The figure shows three views and two pictorial views of one solid part (mm, origin at its lowest corner). Answer the questions. A direction names the side the tool comes from. Round coordinates to 2 decimals unless told otherwise and drop trailing zeros. Order: outer loops, then holes, each group sorted by start corner. A loop starts at its lowest first (then second) coordinate and runs counter-clockwise, first axis right, second up. Notation, with made-up numbers: (41, 28.25) - (49, 28.25) arc R22 cw to (49, 56.25) - close; hole circle Ø5 at (47, 82). An arc over 180 degrees is marked (long way). Use CSV: the item, a comma, the result in double quotes. Start each with the question number.
Item 1: Find section D-D, the plane x = 8.5. Give the vertices of the cut face in (y, z), plus the area to 3 significant figures.
Item 2: Straight lines are drawn through the part: line 1 along X through (y, z) = (0.8, 7.5) (3 decimals); line 2 along Y through (x, z) = (3.25, 3.25); line 3 along Y through (x, z) = (6, 0.6) (3 decimals). For each, find the intervals that lie inside material, in ascending order. Write a range as [from, to].
Item 3: For the marked faces 1 and 2, determine the directions among +Z, -Z, +X, -X, +Y, -Y from which every point of the face is accessible in a straight line to the end or side of a thin tool.
Item 4: Find section C-C, the plane x = 6. Give the vertices of the cut face in (y, z) (3 decimals).
Item 5: Find section A-A, the plane y = 7. Give the vertices of the cut face in (x, z) (3 decimals), plus the area to 3 significant figures.
Item 6: Flat-ended cylindrical pins translate along their axes: P1, Ø3, axis at x = 12, z = 7.5, coming from the +Y side; P2, Ø2, axis at x = 13, y = 5.5, coming from the +Z side. Find the tip coordinate at first contact, or state that the pin passes through.
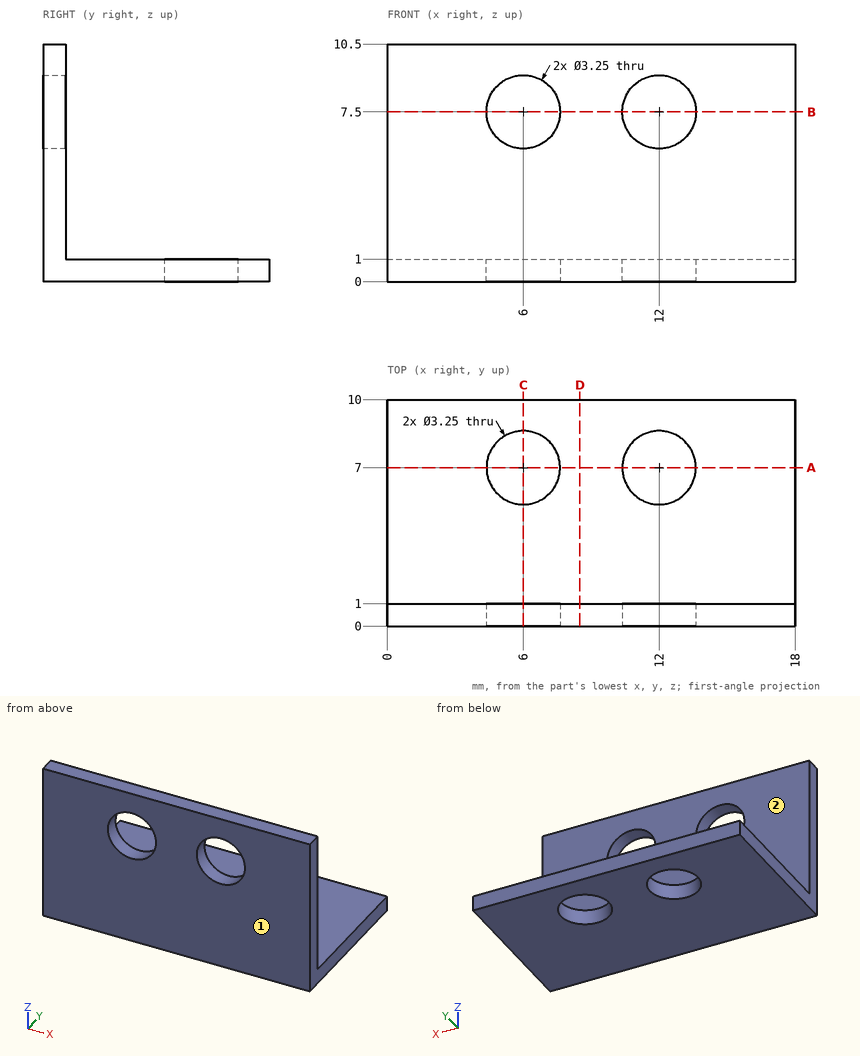
Worked out:
1,outline,"(0, 0) - (10, 0) - (10, 1) - (1, 1) - (1, 10.5) - (0, 10.5) - close"
1,area,"19.5 mm²"
2,line 1,"x = [0, 4.375], [7.625, 10.375], [13.625, 18]"
2,line 2,"y = [0, 1]"
2,line 3,"y = [0, 5.375], [8.625, 10]"
3,face 1,"+Z, -Z, +X, -X, -Y"
3,face 2,"+Z, +X, -X, +Y"
4,outline,"(0, 0) - (5.375, 0) - (5.375, 1) - (1, 1) - (1, 5.875) - (0, 5.875) - close; (0, 9.125) - (1, 9.125) - (1, 10.5) - (0, 10.5) - close; (8.625, 0) - (10, 0) - (10, 1) - (8.625, 1) - close"
5,outline,"(0, 0) - (4.375, 0) - (4.375, 1) - (0, 1) - close; (7.625, 0) - (10.375, 0) - (10.375, 1) - (7.625, 1) - close; (13.625, 0) - (18, 0) - (18, 1) - (13.625, 1) - close"
5,area,"11.5 mm²"
6,P1,"passes through"
6,P2,"stops at z = 1"
